from build123d import *

# Parameters (mm, degrees)
SKETCH030_W             = 51
SKETCH030_H             = 2
SKETCH030_W_2           = 2
SKETCH030_H_2           = 51
PAD018_DEPTH            = 1.5
SKETCH031_R             = 4
SKETCH031_R_2           = 1.6
PAD019_DEPTH            = 2.7
HOLE_D                  = 3.4
HOLE_DEPTH              = 25
HOLE_CSINK_D            = 6.7
HOLE_CSINK_ANGLE        = 90
BODY008_PLACEMENT_ANGLE = 180


with BuildPart() as part:
    # Sketch030 → Pad018 (new body)
    with BuildSketch(Plane.XY):
        with BuildLine():
            Line((-53.5, 40), (-53.5, -42))
            ThreePointArc((-53.5, -42), (-52.328427, -44.828427), (-49.5, -46))
            Line((-49.5, -46), (49.5, -46))
            ThreePointArc((49.5, -46), (52.328427, -44.828427), (53.5, -42))
            Line((53.5, -42), (53.5, 40))
            ThreePointArc((53.5, 40), (52.328427, 42.828427), (49.5, 44))
            Line((49.5, 44), (-49.5, 44))
            ThreePointArc((-49.5, 44), (-52.328427, 42.828427), (-53.5, 40))
        make_face()
        with Locations((0, 34)):
            Rectangle(SKETCH030_W, SKETCH030_H, mode=Mode.SUBTRACT)
        with Locations((0, -34)):
            Rectangle(SKETCH030_W, SKETCH030_H, mode=Mode.SUBTRACT)
        with Locations((36, 0)):
            Rectangle(SKETCH030_W_2, SKETCH030_H_2, mode=Mode.SUBTRACT)
        with Locations((-36, 0)):
            Rectangle(SKETCH030_W_2, SKETCH030_H_2, mode=Mode.SUBTRACT)
    extrude(amount=PAD018_DEPTH)

    # Sketch031 → Pad019 (join)
    with BuildSketch(Plane.XY):
        with Locations((-48.5, 40)):
            Circle(SKETCH031_R)
        with Locations((-48.5, 40)):
            Circle(SKETCH031_R_2, mode=Mode.SUBTRACT)
        with Locations((-30, 40)):
            Circle(SKETCH031_R)
        with Locations((-30, 40)):
            Circle(SKETCH031_R_2, mode=Mode.SUBTRACT)
        with Locations((30, 40)):
            Circle(SKETCH031_R)
        with Locations((30, 40)):
            Circle(SKETCH031_R_2, mode=Mode.SUBTRACT)
        with Locations((30, -41)):
            Circle(SKETCH031_R)
        with Locations((30, -41)):
            Circle(SKETCH031_R_2, mode=Mode.SUBTRACT)
        with Locations((-30, -41)):
            Circle(SKETCH031_R)
        with Locations((-30, -41)):
            Circle(SKETCH031_R_2, mode=Mode.SUBTRACT)
        with Locations((-48.5, -41)):
            Circle(SKETCH031_R)
        with Locations((-48.5, -41)):
            Circle(SKETCH031_R_2, mode=Mode.SUBTRACT)
        with Locations((48.5, -41)):
            Circle(SKETCH031_R)
        with Locations((48.5, -41)):
            Circle(SKETCH031_R_2, mode=Mode.SUBTRACT)
        with Locations((48.5, 40)):
            Circle(SKETCH031_R)
        with Locations((48.5, 40)):
            Circle(SKETCH031_R_2, mode=Mode.SUBTRACT)
    extrude(amount=PAD019_DEPTH)

    # Hole
    with Locations(Plane(origin=(0, 0, 0), x_dir=(1, 0, 0), z_dir=(0, 0, -1))):
        with Locations((-48.5, -40), (-30, -40), (30, -40), (30, 41), (-30, 41), (-48.5, 41), (-48.5, 41), (-30, 41), (30, 41), (30, -40), (-30, -40), (-48.5, -40), (48.5, 41), (48.5, 41), (48.5, -40), (48.5, -40)):
            CounterSinkHole(HOLE_D / 2, HOLE_CSINK_D / 2, depth=HOLE_DEPTH, counter_sink_angle=HOLE_CSINK_ANGLE)


with BuildPart() as part_1:
    # Body008 placement: moved
    add(part.part.moved(Location((0, -1.8, 71.3))).rotate(Axis((0, -1.8, 71.3), (1, 0, 0)), BODY008_PLACEMENT_ANGLE))


solid = part_1.part
Work out the finished part from the listing and answer in its coordinate system (mm). A direction names the side the tool comes from. Give positions to 0.01 mm unless a question says otherwise; leave off trailing zeros. Write each loop counter-clockwise with the first axis right and the second up, starting at its lowest first coordinate (ties: lowest second). Pieces come first, ordered by that corner, then holes. Notation, with made-up numbers: (-8.75, -11.75) - (25.25, -11.75) arc R26 ccw to (25.25, 4.25) - close; hole circle Ø9 at (25, 24). An arc over 180 degrees is marked (long way). One line per item, written item: value. Start each with the question number.
1. Find section B-B (y = -8). Write down the section's boundary in (x, z).
2. Find section A-A (z = 69.2). State how many separate pieces and enclosed holes the cut face has, then the cut area to 3 significant figures.
3. For a pull along X with two mould halves and no side action, classify faces 1 (the cylindrical face through (52.297, 43.059, 70.56)), 2 (the cylindrical face through (-30.521, 35.234, 69.208)), 3 (the flat face through (48, -40, 68.6)) as +X half, -X half, draft (parallel to the pull), parting line (faces both ways), or undercut.
4. For faces 4 (the cylindrical face through (29.479, 35.234, 69.208)), 5 (the cylindrical face through (-47.15, 38.17, 69.12)), determine the directions among +Z, -Z, +X, -X, +Y, -Y from which every point of the face is accessible in a straight line to the end or side of a thin tool.
5. Consider probe 1 along X at (y, z) = (-23.5, 70); probe 2 along Y at (x, z) = (48.5, 69.2); probe 3 along Y at (x, z) = (4, 70.5). Determine where each line is inside the solid, lowest interval first.
6. Given pin 1 (10 mm diameter, centred on x = -13, y = -19.5, fed in from -Z), flat-ended and moving along its own axis, determine where the tip first touches the part or whether it passes through.
7. Find section C-C (x = 14). Write down the section's boundary in (y, z).
Geometry results:
1. outline: (-53.5, 69.8) - (-37, 69.8) - (-37, 71.3) - (-53.5, 71.3) - close; (-35, 69.8) - (35, 69.8) - (35, 71.3) - (-35, 71.3) - close; (37, 69.8) - (53.5, 69.8) - (53.5, 71.3) - (37, 71.3) - close
2. separate pieces: 8
2. enclosed holes: 8
2. area: 329 mm2
3. face 1: +X half
3. face 2: undercut
3. face 3: draft
4. face 4: -Z
4. face 5: +Z, -Z
5. probe 1: -53.5 to -37, -35 to 35, 37 to 53.5
5. probe 2: -45.8 to -43.5, -40.1 to -37.8, 35.2 to 37.5, 40.9 to 43.2
5. probe 3: -45.8 to -36.8, -34.8 to 31.2, 33.2 to 44.2
6. pin 1: z = 69.8
7. outline: (-45.8, 69.8) - (-36.8, 69.8) - (-36.8, 71.3) - (-45.8, 71.3) - close; (-34.8, 69.8) - (31.2, 69.8) - (31.2, 71.3) - (-34.8, 71.3) - close; (33.2, 69.8) - (44.2, 69.8) - (44.2, 71.3) - (33.2, 71.3) - close
